Autodesk Fusion 360 part; units mm, degrees
sketch "Sketch1" plane through (0, 0, 0) normal (0, 0, 1) x (1, 0, 0)
  line L0 (0, 0) -> (8, 0)
  line L1 (8, 0) -> (8, 3.5)
  line L2 (8, 3.5) -> (2, 3.5)
  line L3 (2, 3.5) -> (2, 14.5)
  line L4 (2, 14.5) -> (0, 14.5)
  line L5 (0, 14.5) -> (0, 0)
revolve "Revolve1" add sketch "Sketch1" angle 360 about axis through (0, 14.5, 0) along (0, -1, 0)
sketch "Sketch2" plane through (0, 3.5, 0) normal (0, 1, 0) x (-1, 0, 0)
  circle A0 centre (0, 0) radius 2
  circle A1 centre (0, 0) radius 8
  circle A2 centre (0, 0) radius 4.5
  line L0 (0, 0) -> (1, 0) construction
  line L1 (1, 0) -> (8, 0) construction
  line L2 (0, 0) -> (0, -0.385) construction
  line L3 (0, -0.385) -> (0, -8) construction
  line L4 (0, 0) -> (-8, 0) construction
  line L5 (0, 0) -> (0, 8) construction
  circle A3 centre (4.5, 0) radius 1.5
extrude "Extrude1" cut sketch "Sketch2" against normal blind 1.75 contours A2 A3 | A2 A3 picked at (4.0029, -0.277) picked at (4.9442, -0.3776)
sketch "Sketch3" plane through (0, 1.75, 0) normal (0, 1, 0) x (-1, 0, 0)
  circle A0 centre (4.5, 0) radius 1.5
  circle A1 centre (4.5, 0) radius 0.75
  dimension "d10" = 1.5
extrude "Extrude2" cut sketch "Sketch3" against normal blind 5 contours A1
pattern_circular "C-Pattern1" count 4 over 360 about axis through (0, 1.75, 0) along (0, 1, 0) of "Extrude1"
pattern_circular "C-Pattern2" count 4 over 360 about axis through (0, 1.75, 0) along (0, 1, 0) of "Extrude2"
Read the model definition and answer for the solid it produces. Units are mm, in the model's axes. A direction names the side the tool comes from. Coordinates: 2 decimals unless noted, no trailing zeros. Loops run counter-clockwise (first coordinate to the right, second up) from the corner with the lowest first, then second, coordinate; pieces in that order, holes last. Notation, with made-up numbers: (55.25, 55) -> (91.25, 55) arc R23 ccw to (91.25, 86) -> close; hole circle Ø2 at (56, -8.75). An arc over 180 degrees is marked (long way). Return JSON: item names as keys, results as strings.
Item 1: Find section A-A (x = 0). Determine the outline of the cut face in (y, z), plus the area to 4 significant figures.
Answers:
{"outline": "(0, -8) -> (3.5, -8) -> (3.5, -6) -> (1.75, -6) -> (1.75, -5.25) -> (0, -5.25) -> close; (0, -3.75) -> (1.75, -3.75) -> (1.75, -3) -> (3.5, -3) -> (3.5, -2) -> (14.5, -2) -> (14.5, 2) -> (3.5, 2) -> (3.5, 3) -> (1.75, 3) -> (1.75, 3.75) -> (0, 3.75) -> close; (0, 5.25) -> (1.75, 5.25) -> (1.75, 6) -> (3.5, 6) -> (3.5, 8) -> (0, 8) -> close", "area": "84.25 mm2"}
Item 2: Flat-ended cylindrical pins translate along their axes: P1, Ø1.8, axis at x = -4.5, z = 0, coming from the +Y side; P2, Ø3.5, axis at x = 0, z = 4, coming from the +Y side; P3, Ø8, axis at x = -4.5, y = 7, coming from the -Z side. Find the tip coordinate at first contact, or state that the pin passes through.
Answers:
{"P1": "stops at y = 1.75", "P2": "stops at y = 3.5", "P3": "stops at z = -7.58"}
Item 3: Find section C-C (z = -4.5). Determine the outline of the cut face in (x, y).
Answers:
{"outline": "(-6.61, 0) -> (-0.75, 0) -> (-0.75, 1.75) -> (-1.5, 1.75) -> (-1.5, 3.5) -> (-6.61, 3.5) -> close; (0.75, 0) -> (6.61, 0) -> (6.61, 3.5) -> (1.5, 3.5) -> (1.5, 1.75) -> (0.75, 1.75) -> close"}
Item 4: Find section B-B (z = -0.5). Determine the outline of the cut face in (x, y), plus the area to 3 significant figures.
Answers:
{"outline": "(-7.98, 0) -> (-5.06, 0) -> (-5.06, 1.75) -> (-5.91, 1.75) -> (-5.91, 3.5) -> (-7.98, 3.5) -> close; (-3.94, 0) -> (3.94, 0) -> (3.94, 1.75) -> (3.09, 1.75) -> (3.09, 3.5) -> (1.94, 3.5) -> (1.94, 14.5) -> (-1.94, 14.5) -> (-1.94, 3.5) -> (-3.09, 3.5) -> (-3.09, 1.75) -> (-3.94, 1.75) -> close; (5.06, 0) -> (7.98, 0) -> (7.98, 3.5) -> (5.91, 3.5) -> (5.91, 1.75) -> (5.06, 1.75) -> close", "area": "84.7 mm2"}
Item 5: Find section D-D (x = 5.75). Determine the outline of the cut face in (y, z).
Answers:
{"outline": "(0, -5.56) -> (3.5, -5.56) -> (3.5, -0.83) -> (1.75, -0.83) -> (1.75, 0.83) -> (3.5, 0.83) -> (3.5, 5.56) -> (0, 5.56) -> close"}
Item 6: For faces 1 (the cylindrical face through (-1.73, 1.77, 7.81)), 2 (the flat face through (2, 3.5, -2)), determine the directions among +Z, -Z, +X, -X, +Y, -Y from which every point of the face is accessible in a straight line to the end or side of a thin tool.
Answers:
{"face 1": "+Y, -Y", "face 2": "+Y"}
Item 7: For a pull along X with two mould halves and no side action, classify faces 3 (the cylindrical face through (0, 9, 2)), 4 (the flat face through (0, 0, 0)), 5 (the flat face through (-1, 1.75, -5)) as +X half, -X half, draft (parallel to the pull), parting line (faces both ways), or undercut.
Answers:
{"face 3": "parting line", "face 4": "draft", "face 5": "undercut"}
Item 8: Find the intervals of material crossed by probe 1 along Z at (x, y) = (0, 2.45); probe 2 along Y at (x, z) = (7.25, -2); probe 3 along Z at (x, y) = (-4.5, 0.95), in increasing order.
Answers:
{"probe 1": "z = -8 to -6, -3 to 3, 6 to 8", "probe 2": "y = 0 to 3.5", "probe 3": "z = -6.61 to -0.75, 0.75 to 6.61"}
